The listing builds one solid part. Answer for the finished solid, in the listing's coordinates (mm). Face numbers are marked on the shaded views. A direction names the side the tool comes from. Round coordinates to 2 decimals unless told otherwise and drop trailing zeros. Write each loop counter-clockwise with the first axis right and the second up, starting at its lowest first coordinate (ties: lowest second). Pieces come first, ordered by that corner, then holes. Notation, with made-up numbers: (10, 27.25) - (68, 27.25) arc R20 ccw to (68, 38.25) - close; hole circle Ø7 at (-19.75, -37.75). An arc over 180 degrees is marked (long way). Use a Markdown table: item, result. Add a question column.
1) A cutting plane is placed at C-C (z = -12). Give the vertices of the cut face in (x, y), then the cut area to 3 significant figures.
2) A tool of negligible diameter and unlimited length cuts with its end or side. For the marked faces 1 and 2, from which of +Z, -Z, +X, -X, +Y, -Y can it reach the whole face along a straight path? Write none if from no direction.
3) A cutting plane is placed at B-B (x = 13.5). Give the vertices of the cut face in (y, z).
4) Find the intervals of material crossed by probe 1 along Z at (x, y) = (55, -9); probe 2 along X at (y, z) = (-9.25, -7.75), in increasing order. Write a range as from..to.
5) Determine the mould class of the marked faces 3, 4 and 5 for opening direction Z: +Z half, -Z half, draft (parallel to the pull), parting line (faces both ways), or undercut.
6) A cutting plane is placed at A-A (y = -22). Give the vertices of the cut face in (x, z), then the cut area to 3 significant figures.
7) Each of these flat-tipped pins is pushed along its axis until it touches: P1, Ø6, axis at y = -14, z = -3.5, coming from the +X side; P2, Ø10, axis at x = 49, y = -12, coming from the -Z side; P3, Ø8, axis at x = 27, z = -5.5, coming from the +Y side; P4, Ø8, axis at x = 40, z = -2, coming from the +Y side. Where does it stop, or does it pass through?
Autodesk Inventor part; units mm, degrees
ref_plane "YZ Plane" through (0, 0, 0) normal (1, 0, 0) x (0, 1, 0)
ref_plane "XZ Plane" through (0, 0, 0) normal (0, 1, 0) x (-1, 0, 0)
ref_plane "XY Plane" through (0, 0, 0) normal (0, 0, 1) x (1, 0, 0)
sketch "Sketch1" plane through (0, 0, 0) normal (0, 0, 1) x (1, 0, 0)
  line L0 (0, 0) -> (63, 0)
  line L1 (63, 0) -> (63, -25)
  line L2 (63, -25) -> (0, -25)
  line L3 (0, -25) -> (0, 0)
  dimension "d0" = 63
  dimension "d1" = 25
extrude "Extrusion1" add sketch "Sketch1" along normal blind 3
sketch "Sketch2" plane through (0, -25, 0) normal (-1, 0, 0) x (0, 0, 1)
  line L0 (3, 0) -> (3, 25)
  line L1 (3, 25) -> (-15, 25)
  line L2 (-15, 25) -> (-15, 0)
  line L3 (-15, 0) -> (3, 0)
  line L4 (3, 0) -> (3, 25)
  point P0 (0, 25)
  dimension "d4" = 18
extrude "Extrusion2" add sketch "Sketch2" along normal blind 3
properties part number "arduino array box v04 slot"
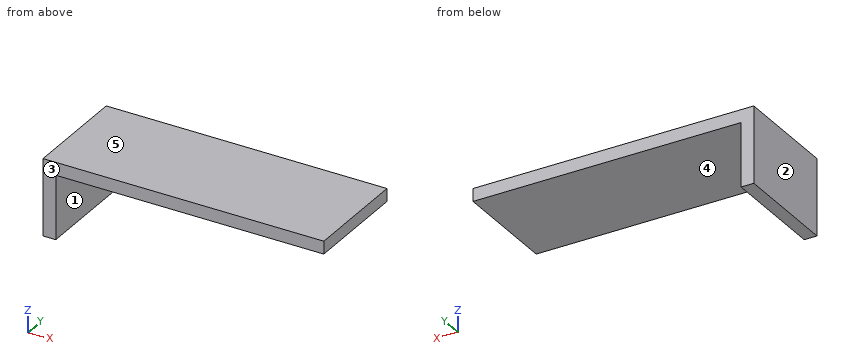
Entries:
| question | item | result |
|---|---|---|
| 1 | outline | (-3, -25) - (0, -25) - (0, 0) - (-3, 0) - close |
| 1 | area | 75.0 mm² |
| 2 | face 1 | -Z, +X, +Y, -Y |
| 2 | face 2 | +Z, -Z, -X, +Y, -Y |
| 3 | outline | (-25, 0) - (0, 0) - (0, 3) - (-25, 3) - close |
| 4 | probe 1 | z = 0..3 |
| 4 | probe 2 | x = -3..0 |
| 5 | face 3 | draft |
| 5 | face 4 | -Z half |
| 5 | face 5 | +Z half |
| 6 | outline | (-3, -15) - (0, -15) - (0, 0) - (63, 0) - (63, 3) - (-3, 3) - close |
| 6 | area | 243 mm² |
| 7 | P1 | stops at x = 0 |
| 7 | P2 | stops at z = 0 |
| 7 | P3 | passes through |
| 7 | P4 | stops at y = 0 |
